from build123d import *

# Parameters (mm, degrees)
SKETCH1_R           = 1.55
SKETCH1_R_2         = 5
SKETCH1_R_3         = 6
BOSS_EXTRUDE1_DEPTH = 3
FILLET1_R           = 3


with BuildPart() as part:
    # Sketch1 → Boss-Extrude1 (new body)
    with BuildSketch(Plane(origin=(0, 0, 0), x_dir=(1, 0, 0), z_dir=(0, 1, 0))):
        Polygon((-62, 19), (62, 19), (62, 13), (59, 13), (59, -13), (62, -13), (62, -19), (-62, -19), (-62, -13), (-59, -13), (-59, 13), (-62, 13), align=None)
        with Locations(Location((55.5, 11, 0), (0, 0, 270))):
            Circle(SKETCH1_R, mode=Mode.SUBTRACT)
        with Locations(Location((-55.5, 11, 0), (0, 0, 90))):
            Circle(SKETCH1_R, mode=Mode.SUBTRACT)
        with Locations(Location((-55.5, -11, 0), (0, 0, 270))):
            Circle(SKETCH1_R, mode=Mode.SUBTRACT)
        with Locations(Location((55.5, -11, 0), (0, 0, 90))):
            Circle(SKETCH1_R, mode=Mode.SUBTRACT)
        with Locations(Location((0, 0, 0), (0, 0, 270))):
            Circle(SKETCH1_R_2, mode=Mode.SUBTRACT)
        with Locations(Location((20, 0, 0), (0, 0, 270))):
            Circle(SKETCH1_R, mode=Mode.SUBTRACT)
        with Locations(Location((-20, 0, 0), (0, 0, 90))):
            Circle(SKETCH1_R, mode=Mode.SUBTRACT)
        with Locations(Location((35, 0, 0), (0, 0, 270))):
            Circle(SKETCH1_R_3, mode=Mode.SUBTRACT)
        with Locations(Location((-35, 0, 0), (0, 0, 90))):
            Circle(SKETCH1_R_3, mode=Mode.SUBTRACT)
        with Locations(Location((47, 9, 0), (0, 0, 270))):
            Circle(SKETCH1_R, mode=Mode.SUBTRACT)
        with Locations(Location((47, -9, 0), (0, 0, 90))):
            Circle(SKETCH1_R, mode=Mode.SUBTRACT)
        with Locations(Location((-47, -9, 0), (0, 0, 270))):
            Circle(SKETCH1_R, mode=Mode.SUBTRACT)
        with Locations(Location((-47, 9, 0), (0, 0, 90))):
            Circle(SKETCH1_R, mode=Mode.SUBTRACT)
    extrude(amount=BOSS_EXTRUDE1_DEPTH)

    # Fillet1
    fillet1_edges = [part.edges().sort_by_distance(p)[0] for p in [
        (-62, 1.5, -19),
        (-62, 1.5, -13),
        (-62, 1.5, 13),
        (-62, 1.5, 19),
        (62, 1.5, 19),
        (62, 1.5, 13),
        (62, 1.5, -13),
        (62, 1.5, -19),
    ]]
    fillet(fillet1_edges, radius=FILLET1_R - 0.0001)  # a hair under: the kernel refuses the full size


solid = part.part
Read the model definition and answer for the solid it produces. Units are mm, in the model's axes. A direction names the side the tool comes from. Round coordinates to 2 decimals unless told otherwise and drop trailing zeros. Write each loop counter-clockwise with the first axis right and the second up, starting at its lowest first coordinate (ties: lowest second). Pieces come first, ordered by that corner, then holes.
Q1. Straight lines are drawn through the part: line 1 (X direction, y = 2.25, z = -11); line 2 (X direction, y = 1.4, z = 0); line 3 (Z direction, x = -20, y = 2.1). For each, find the intervals that lie inside material, in ascending order.
Values:
line 1: x = -59 to -57.05, -53.95 to 53.95, 57.05 to 59
line 2: x = -59 to -41, -29 to -21.55, -18.45 to -5, 5 to 18.45, 21.55 to 29, 41 to 59
line 3: z = -19 to -1.55, 1.55 to 19
Q2. Find section B-B on x = -55.5. Determine the outline of the cut face in (y, z), and give its area (3 significant figures).
Values:
outline: (0, -19) - (3, -19) - (3, -12.55) - (0, -12.55) - close; (0, -9.45) - (3, -9.45) - (3, 9.45) - (0, 9.45) - close; (0, 12.55) - (3, 12.55) - (3, 19) - (0, 19) - close
area: 95.4 mm2
Q3. Flat-ended cylindrical pins translate along their axes: P1, Ø0.9, axis at y = 1, z = -4, coming from the +X side; P2, Ø4, axis at x = 47, z = -9, coming from the -Y side; P3, Ø1.5, axis at y = 2.5, z = -10.5, coming from the -X side. Find the tip coordinate at first contact, or state that the pin passes through.
Values:
P1: stops at x = 59
P2: stops at y = 0
P3: stops at x = -59
Q4. A tool of negligible diameter and unlimited length cuts with its end or side. For faces 1 (the face through (-59, 1, 0)), 2 (the face through (-4.88, 1.48, -1.08)), 3 (the face through (61.14, 1.52, -13.9)), from which of +Z, -Z, +X, -X, +Y, -Y can it reach the whole face along a straight path? Write none if from no direction.
Values:
face 1: -X, +Y, -Y
face 2: +Y, -Y
face 3: +X, +Y, -Y
Q5. Find section C-C on z = -3.5. Determine the outline of the cut face in (x, y), and give its area (3 significant figures).
Values:
outline: (-59, 0) - (-39.87, 0) - (-39.87, 3) - (-59, 3) - close; (-30.13, 0) - (-3.57, 0) - (-3.57, 3) - (-30.13, 3) - close; (3.57, 0) - (30.13, 0) - (30.13, 3) - (3.57, 3) - close; (39.87, 0) - (59, 0) - (59, 3) - (39.87, 3) - close
area: 274 mm2
Q6. The mould has two halves that part along Z. Classify faces 4 (the face through (1, 1, 19)), 5 (the face through (-1, 1, -19)), 6 (the face through (59, 1, 0)): released by +Z, released by -Z, zero draft, split by the parting line, or undercut.
Values:
face 4: released by +Z
face 5: released by -Z
face 6: undercut
Q7. Find section D-D on y = 0.85. State how many separate pieces and enclosed holes the cut face has, and give its area (3 significant figures).
Values:
separate pieces: 1
enclosed holes: 13
area: 4,160 mm2
Q8. Find section A-A on x = 0. Determine the outline of the cut face in (y, z), and give its area (3 significant figures).
Values:
outline: (0, -19) - (3, -19) - (3, -5) - (0, -5) - close; (0, 5) - (3, 5) - (3, 19) - (0, 19) - close
area: 84.0 mm2
